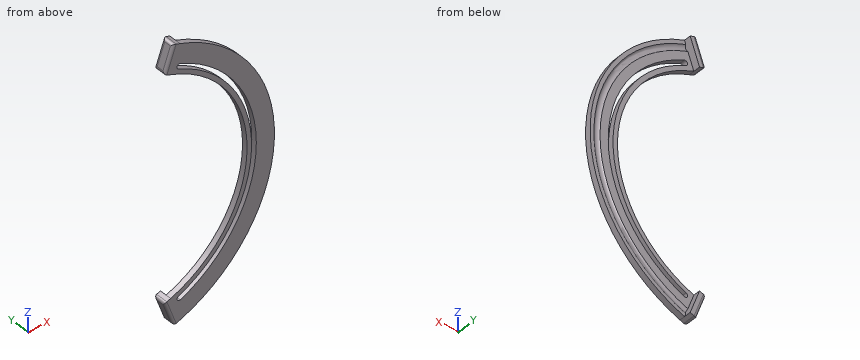
from build123d import *

# Parameters (mm, degrees)
REVOLVE_1_ANGLE     = 140
SKETCH_3_W          = 20
SKETCH_3_H          = 9
EXTRUDE_1_DEPTH     = 5
SKETCH_4_W          = 20
SKETCH_4_H          = 9
EXTRUDE_2_DEPTH     = 5
CUT_EXTRUDE_1_DEPTH = 5
FILLET_1_R          = 2


with BuildPart() as part:
    # 草图2 → 旋转1 (revolve, symmetric)
    with BuildSketch(Plane.XY) as revolve_1_sk:
        with BuildLine():
            ThreePointArc((102.236067977, -6), (100, -7), (97.763932023, -6))
            Line((97.763932023, -6), (85, -6))
            Line((85, -6), (85, -10))
            Line((85, -10), (105, -10))
            Line((105, -10), (105, -6))
            Line((105, -6), (102.236067977, -6))
        make_face()
    revolve(axis=Axis((0, 24.366902053, 0), (0, -1, 0)), revolution_arc=REVOLVE_1_ANGLE / 2)
    revolve(revolve_1_sk.sketch, axis=Axis((0, 24.366902053, 0), (0, 1, 0)), revolution_arc=REVOLVE_1_ANGLE / 2)

    # 草图3 → 凸台-拉伸1 (add)
    with BuildSketch(Plane(origin=(0, 0, 0), x_dir=(0.34202014332566616, 0, 0.9396926207859094), z_dir=(-0.9396926207859093, 0, 0.3420201433256661))):
        with Locations((95, -5.5)):
            Rectangle(SKETCH_3_W, SKETCH_3_H)
    extrude(amount=EXTRUDE_1_DEPTH)

    # 草图4 → 凸台-拉伸2 (add)
    with BuildSketch(Plane(origin=(0, 0, 0), x_dir=(-0.34202014332566616, 0, 0.9396926207859094), z_dir=(-0.9396926207859094, 0, -0.34202014332566616))):
        with Locations((-95, -5.5)):
            Rectangle(SKETCH_4_W, SKETCH_4_H)
    extrude(amount=EXTRUDE_2_DEPTH)

    # 草图5 → 切除-拉伸1 (cut)
    with BuildSketch(Plane(origin=(0, -6, 0), x_dir=(1, 0, 0), z_dir=(0, 1, 0))):
        with BuildLine():
            ThreePointArc((34.743766956, 81.122950869), (88.25, -6.1e-08), (34.743766843, -81.122950917))
            ThreePointArc((34.743766843, -81.122950917), (33.82406612, -83.420591403), (36.121706789, -84.340291668))
            ThreePointArc((36.121706789, -84.340291668), (91.75, 4e-08), (36.121706715, 84.3402917))
            ThreePointArc((36.121706715, 84.3402917), (33.82406608, 83.42059131), (34.743766956, 81.122950869))
        make_face()
    extrude(amount=-CUT_EXTRUDE_1_DEPTH, mode=Mode.SUBTRACT)

    # 圆角1
    fillet_1_edges = [part.edges().sort_by_distance(p)[0] for p in [
        (24.373249079, -5.5, 81.583973483),
        (31.213651945, -5.5, 100.377825899),
        (27.793450512, -1, 90.980899691),
        (27.793450512, -10, 90.980899691),
        (31.213651945, -5.5, -100.377825899),
        (24.373249079, -5.5, -81.583973483),
        (27.793450512, -1, -90.980899691),
        (27.793450512, -10, -90.980899691),
    ]]
    fillet(fillet_1_edges, radius=FILLET_1_R)


solid = part.part
The listing builds one solid part. Answer for the finished solid, in the listing's coordinates (mm). Coordinates: 2 decimals unless noted, no trailing zeros. Answer in a Markdown table with one row per item.
1) Find section A-A (x = 39.5). Count the separate pieces of the cut face and the enclosed holes in it, then the cut area to 3 significant figures.
Answers below:
| item | result |
|---|---|
| separate pieces | 4 |
| enclosed holes | 0 |
| area | 138 mm^2 |
2) Given pin 1 (20.5 mm diameter, centred on x = 61, z = -23.5, fed in from +Y); pin 2 (1.5 mm diameter, centred on x = 86, y = -8.5, fed in from -Z); pin 3 (3 mm diameter, centred on x = 76.5, z = -34.5, fed in from +Y); pin 4 (1.5 mm diameter, centred on x = 79, y = -5.5, fed in from -Z), each flat-ended and moving along its own axis, determine where each tip first touches the part or whether it passes through.
Answers below:
| item | result |
|---|---|
| pin 1 | through |
| pin 2 | z = -61.3 |
| pin 3 | y = -6 |
| pin 4 | z = -69.8 |
3) Find the intervals of material crossed by probe 1 along Z at (x, y) = (38.5, -7.25); probe 2 along Z at (x, y) = (45, -9.25); probe 3 along X at (y, z) = (-8.5, -31), in increasing order.
Answers below:
| item | result |
|---|---|
| probe 1 | -97.69 to -83.28, -79.41 to -75.78, 75.78 to 79.41, 83.28 to 97.69 |
| probe 2 | -94.87 to -79.96, -75.91 to -72.11, 72.11 to 75.91, 79.96 to 94.87 |
| probe 3 | 79.15 to 82.63, 86.35 to 100.32 |
